from build123d import *

# Parameters (mm, degrees)
BOSS_EXTRUDE1_DEPTH = 25
CUT_EXTRUDE1_DEPTH  = 85
SKETCH3_W           = 36
SKETCH3_H           = 16
BOSS_EXTRUDE2_DEPTH = 13
SKETCH4_R           = 6
CUT_EXTRUDE2_DEPTH  = 23
BOSS_EXTRUDE3_DEPTH = 13
CUT_EXTRUDE4_REACH  = 110.497
SKETCH7_R           = 2.1
CUT_EXTRUDE5_DEPTH  = 11.5
SKETCH10_R          = 4.1
CUT_EXTRUDE6_DEPTH  = 114.014379616
SKETCH11_R          = 4.1
CUT_EXTRUDE7_DEPTH  = 6.4
FILLET1_R           = 5


with BuildPart() as part:
    # Sketch1 → Boss-Extrude1 (new body)
    with BuildSketch(Plane(origin=(0, 0, 0), x_dir=(1, 0, 0), z_dir=(0, 1, 0))):
        with BuildLine():
            Line((0, -22.5), (-105, -22.5))
            Line((-105, -22.5), (-105, 22.5))
            Line((-105, 22.5), (0, 22.5))
            ThreePointArc((0, 22.5), (11.374313166, 19.413268658), (19.627786426, 11))
            Line((19.627786426, 11), (38, 11))
            Line((38, 11), (38, 1))
            Line((38, 1), (22, 1))
            Line((22, 1), (12.610412364, 1))
            ThreePointArc((12.610412364, 1), (-12.65, 0), (12.610412364, -1))
            Line((12.610412364, -1), (22, -1))
            Line((22, -1), (38, -1))
            Line((38, -1), (38, -11))
            Line((38, -11), (19.627786426, -11))
            ThreePointArc((19.627786426, -11), (11.374313166, -19.413268658), (0, -22.5))
        make_face()
    extrude(amount=BOSS_EXTRUDE1_DEPTH)

    # Sketch2 → Cut-Extrude1 (cut)
    with BuildSketch(Plane.ZY.offset(105)):
        Polygon((20, 25), (-20, 25), (-22.5, 25), (-22.5, 15.5), (-20, 15.5), (-20, 2.5), (20, 2.5), (20, 15.5), (22.5, 15.5), (22.5, 25), align=None)
    extrude(amount=-CUT_EXTRUDE1_DEPTH, mode=Mode.SUBTRACT)

    # Sketch3 → Boss-Extrude2 (add)
    with BuildSketch(Plane(origin=(0, 2.5, 0), x_dir=(1, 0, 0), z_dir=(0, 1, 0))):
        with Locations((-87, 0)):
            Rectangle(SKETCH3_W, SKETCH3_H)
    extrude(amount=BOSS_EXTRUDE2_DEPTH)

    # Sketch4 → Cut-Extrude2 (cut)
    with BuildSketch(Plane(origin=(-69, 0, 0), x_dir=(0, 0, -1), z_dir=(1, 0, 0))):
        with Locations((0, 9)):
            Circle(SKETCH4_R)
    extrude(amount=-CUT_EXTRUDE2_DEPTH, mode=Mode.SUBTRACT)

    # Sketch6 → Boss-Extrude3 (add)
    with BuildSketch(Plane(origin=(0, 2.5, 0), x_dir=(1, 0, 0), z_dir=(0, 1, 0))):
        Polygon((-35, -20), (-20, -5), (-20, -20), align=None)
        Polygon((-20, 20), (-20, 5), (-35, 20), align=None)
    extrude(amount=BOSS_EXTRUDE3_DEPTH)

    # Sketch7 → Cut-Extrude4 (cut, up to next)
    with BuildSketch(Plane(origin=(0, 15.5, 0), x_dir=(1, 0, 0), z_dir=(0, 1, 0)), mode=Mode.PRIVATE) as cut_extrude4_sk1:
        with Locations(Location((-25, -17.5, 0), (0, 0, 270))):
            Circle(SKETCH7_R)
    cut_extrude4_tool1 = extrude(cut_extrude4_sk1.sketch, amount=-CUT_EXTRUDE4_REACH, mode=Mode.PRIVATE) & part.part
    # Sketch7 → Cut-Extrude4 (cut, up to next)
    with BuildSketch(Plane(origin=(0, 15.5, 0), x_dir=(1, 0, 0), z_dir=(0, 1, 0)), mode=Mode.PRIVATE) as cut_extrude4_sk2:
        with Locations(Location((-25, 17.5, 0), (0, 0, 270))):
            Circle(SKETCH7_R)
    cut_extrude4_tool2 = extrude(cut_extrude4_sk2.sketch, amount=-CUT_EXTRUDE4_REACH, mode=Mode.PRIVATE) & part.part
    # Sketch7 → Cut-Extrude4 (cut, up to next)
    with BuildSketch(Plane(origin=(0, 15.5, 0), x_dir=(1, 0, 0), z_dir=(0, 1, 0)), mode=Mode.PRIVATE) as cut_extrude4_sk3:
        with Locations(Location((-99, 0, 0), (0, 0, 270))):
            Circle(SKETCH7_R)
    cut_extrude4_tool3 = extrude(cut_extrude4_sk3.sketch, amount=-CUT_EXTRUDE4_REACH, mode=Mode.PRIVATE) & part.part
    add(cut_extrude4_tool1.solids().sort_by_distance((-25, 15.5, 17.5))[0], mode=Mode.SUBTRACT)
    add(cut_extrude4_tool2.solids().sort_by_distance((-25, 15.5, -17.5))[0], mode=Mode.SUBTRACT)
    add(cut_extrude4_tool3.solids().sort_by_distance((-99, 15.5, 0))[0], mode=Mode.SUBTRACT)

    # Sketch8 → Cut-Extrude5 (cut)
    with BuildSketch(Plane(origin=(0, 0, 0), x_dir=(-1, 0, 0), z_dir=(0, -1, 0))):
        Polygon((20.843078062, 17.5), (22.921539031, 13.9), (27.078460969, 13.9), (29.156921938, 17.5), (27.078460969, 21.1), (22.921539031, 21.1), align=None)
        Polygon((20.843078062, -17.5), (22.921539031, -21.1), (27.078460969, -21.1), (29.156921938, -17.5), (27.078460969, -13.9), (22.921539031, -13.9), align=None)
        Polygon((99, -4.156921938), (102.6, -2.078460969), (102.6, 2.078460969), (99, 4.156921938), (95.4, 2.078460969), (95.4, -2.078460969), align=None)
    extrude(amount=-CUT_EXTRUDE5_DEPTH, mode=Mode.SUBTRACT)

    # Sketch10 → Cut-Extrude6 (cut, through all)
    with BuildSketch(Plane.XY.offset(11)):
        with Locations((29, 12.5)):
            Circle(SKETCH10_R)
    extrude(amount=-CUT_EXTRUDE6_DEPTH, mode=Mode.SUBTRACT)

    # Sketch11 → Cut-Extrude7 (cut)
    with BuildSketch(Plane(origin=(0, 0, 11), x_dir=(-1, 0, 0), z_dir=(0, 0, -1))):
        Polygon((-35.6, 16.310511777), (-35.6, 8.689488223), (-29, 4.878976447), (-22.4, 8.689488223), (-22.4, 16.310511777), (-29, 20.121023553), align=None)
        with Locations(Location((-29, 12.5, 0), (0, 0, 180))):
            Circle(SKETCH11_R, mode=Mode.SUBTRACT)
    extrude(amount=CUT_EXTRUDE7_DEPTH, mode=Mode.SUBTRACT)

    # Fillet1
    fillet1_edges = [part.edges().sort_by_distance(p)[0] for p in [
        (38, 25, 6),
        (38, 0, -6),
        (38, 0, 6),
        (38, 25, -6),
    ]]
    fillet(fillet1_edges, radius=FILLET1_R)


solid = part.part
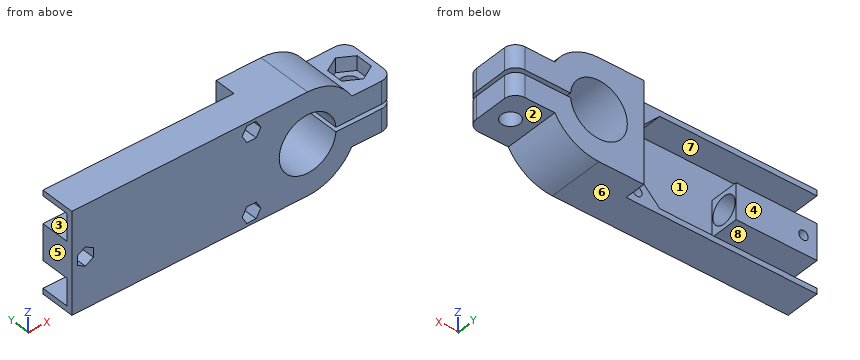
Work out the finished part from the listing and answer in its coordinate system (mm). Face numbers are marked on the shaded views. A direction names the side the tool comes from. Round coordinates to 2 decimals unless told otherwise and drop trailing zeros. Order: outer loops, then holes, each group sorted by start corner. A loop starts at its lowest first (then second) coordinate and runs counter-clockwise, first axis right, second up. Notation, with made-up numbers: M 1,-5.5 L 6,-5.5 A28 ccw 6,32.5 Z; hole C -26,87.25 d5. An arc over 180 degrees is marked long. One line per item, written item: value.
Q1. Find section D-D on x = -33. Write down the section's boundary in (y, z).
Derived:
outline: M 0,-22.5 L 15.5,-22.5 L 15.5,-18 L 2.5,-18 L 2.5,18 L 15.5,18 L 15.5,22.5 L 0,22.5 Z
Q2. Flat-ended cylindrical pins translate along their axes: pin 1 (5 mm diameter, centred on y = 16.5, z = 17.5, fed in from -X); pin 2 (8 mm diameter, centred on x = -31, z = -2.5, fed in from -Y); pin 3 (2 mm diameter, centred on y = 6, z = 17.5, fed in from -X); pin 4 (19 mm diameter, centred on x = -70.5, z = 11, fed in from +Y). Find the tip coordinate at first contact, or state that the pin passes through.
Derived:
pin 1: x = -34.79
pin 2: y = 0
pin 3: x = -33.5
pin 4: y = 15.5
Q3. Find section A-A on x = -61. Write down the section's boundary in (y, z).
Derived:
outline: M 0,-22.5 L 15.5,-22.5 L 15.5,-20 L 2.5,-20 L 2.5,20 L 15.5,20 L 15.5,22.5 L 0,22.5 Z
Q4. Straight lines are drawn through the part: line 1 (X direction, y = 13.3, z = 0); line 2 (Y direction, x = 29, z = -4); line 3 (X direction, y = 15.75, z = -5.5). For each, find the intervals that lie inside material, in ascending order.
Derived:
line 1: -105 to -101.1, -96.9 to -92, -20 to -12.65
line 2: 0 to 8.4, 16.6 to 25
line 3: -20 to -11.39, 11.39 to 26.5, 31.5 to 38
Q5. For the marked faces 1, 2, 3 and 4, determine the directions among +Z, -Z, +X, -X, +Y, -Y from which every point of the face is accessible in a straight line to the end or side of a thin tool.
Derived:
face 1: +Y
face 2: -Z, +X, +Y, -Y
face 3: -X, +Y
face 4: +Z, -Z, -X, +Y
Q6. Determine the mould class of the marked faces 5, 6, 7 and 8 for opening direction Z: released by +Z, released by -Z, zero draft, split by the parting line, or undercut.
Derived:
face 5: zero draft
face 6: released by -Z
face 7: undercut
face 8: undercut
Q7. Find section C-C on y = 23.25. Write down the section's boundary in (x, z).
Derived:
outline: M -20,-22.5 L 0,-22.5 A22.5 ccw 19.63,-11 L 36.8,-11 L 36.8,-1 L 12.61,-1 A12.65 cw long 12.61,1 L 36.8,1 L 36.8,11 L 19.63,11 A22.5 ccw 0,22.5 L -20,22.5 Z
Q8. Find section B-B on x = 16.5. Write down the section's boundary in (y, z), then the cut area to 3 significant figures.
Derived:
outline: M 0,-15.3 L 25,-15.3 L 25,-1 L 0,-1 Z; M 0,1 L 25,1 L 25,15.3 L 0,15.3 Z
area: 715 mm²
